Geometry check sheet. Reference: the model listing, model coordinates, mm. A direction names the side the tool comes from. Coordinates: 2 decimals unless noted, no trailing zeros. Loops run counter-clockwise (first coordinate to the right, second up) from the corner with the lowest first, then second, coordinate; pieces in that order, holes last.
Autodesk Inventor part; units mm, degrees
ref_plane "YZ Plane" through (0, 0, 0) normal (1, 0, 0) x (0, 1, 0)
ref_plane "XZ Plane" through (0, 0, 0) normal (0, 1, 0) x (-1, 0, 0)
ref_plane "XY Plane" through (0, 0, 0) normal (0, 0, 1) x (1, 0, 0)
sketch "Sketch1" plane through (0, 0, 0) normal (0, 0, 1) x (1, 0, 0)
  line L0 (0, 0) -> (0, 15)
  line L1 (0, 0) -> (15, 0)
  arc A0 (15, 0) -> (0, 15) centre (0, 0) ccw
  line L2 (0, -3.6213) -> (0, 21.7279)
  dimension "d2" = 15
revolve "Revolution1" add sketch "Sketch1" angle 360 about axis through (0, -10, 0) along (0, 1, 0)
sketch "Sketch4" plane through (0, 0, 0) normal (0, -1, 0) x (1, 0, 0)
  point P0 (0, 0)
  point P1 (0, 0)
hole "Hole2" at (0, 0, 0) direction (0, 1, 0) diameter 3.242 depth 11.8 tip angle 118
shell "Shell2" thickness 5 removed faces 1 at (10.3911, 0, 1.2617)
properties part number "Ball_Upper Half" material "Nylon 6/6"
1) Section check C-C on y = 8.25. Record the cut outline in (x, z).
Data:
outline: circle Ø25.05 at (0, 0); hole circle Ø3.24 at (0, 0)
2) Mould release check, pull along Z, two halves, no side actions. Record for faces 1 (the flat face through (-3, 0, 10)), 2 (the cylindrical face through (6.464, 3.8, 1.435)): +Z half, -Z half, draft (parallel to the pull), parting line (faces both ways), or undercut.
Data:
face 1: draft
face 2: undercut
3) Material ranges on probe 1 along Z at (x, y) = (3, 3.5); probe 2 along Z at (x, y) = (-5.75, 7); probe 3 along Z at (x, y) = (0, 7), recorded low to high.
Data:
probe 1: z = -14.27 to -8.87, -5.9 to 5.9, 8.87 to 14.27
probe 2: z = -11.96 to -4.24, -3.28 to 3.28, 4.24 to 11.96
probe 3: z = -13.27 to -7.14, -6.62 to -1.62, 1.62 to 6.62, 7.14 to 13.27
4) Depth check by flat-ended pin: pin 1 (2 mm diameter, centred on y = 8.5, z = -8.5, fed in from -X); pin 2 (6 mm diameter, centred on x = 8, z = 10.5, fed in from -Y); pin 3 (8 mm diameter, centred on y = 12.5, z = 5.5, fed in from +X); pin 4 (8 mm diameter, centred on y = 2.5, z = -8, fed in from +X). Enter the tip coordinate at first touch or a pass-through.
Data:
pin 1: stops at x = -10.18
pin 2: stops at y = 0
pin 3: stops at x = 11.48
pin 4: stops at x = 14.35
5) Section check D-D on x = 8. Record the cut outline in (y, z).
Data:
outline: (0, -12.69) arc R12.69 ccw to (0, 12.69) - (0, 6) arc R6 cw to (0, -6) - close
6) Section check A-A on y = 5.5. Record the cut outline in (x, z).
Data:
outline: circle Ø27.91 at (0, 0); circle Ø13.24 at (0, 0); hole circle Ø16.7 at (0, 0); hole circle Ø3.24 at (0, 0)
7) Section check B-B on z = -3.5. Record the cut outline in (x, y) (1 decimal), and give its area (3 significant figures).
Data:
outline: (-14.6, 0) - (-9.4, 0) arc R9.4 cw to (-5.6, 7.5) - (-5.6, 0) - (5.6, 0) - (5.6, 7.5) arc R9.4 cw to (9.4, 0) - (14.6, 0) arc R14.6 ccw to start
area: 295 mm2
8) Access from +Z, -Z, +X, -X, +Y, -Y to the whole of each face (thin tool, end or side, straight path). Record for faces 3 (the flat face through (-1.4, 0, 1.4)), 4 (the cylindrical face through (1.438, 5.983, -0.748)).
Data:
face 3: +Z, -Z, +X, -X, -Y
face 4: -Y
